Autodesk Inventor part; units mm, degrees
ref_plane "YZ Plane" through (0, 0, 0) normal (1, 0, 0) x (0, 1, 0)
ref_plane "XZ Plane" through (0, 0, 0) normal (0, 1, 0) x (-1, 0, 0)
ref_plane "XY Plane" through (0, 0, 0) normal (0, 0, 1) x (1, 0, 0)
sketch "Sketch1" plane through (0, 0, 0) normal (0, 0, 1) x (1, 0, 0)
  circle A0 centre (0, 0) radius 12.2
  dimension "d0" = 24.4
extrude "Extrusion1" add sketch "Sketch1" along normal blind 34
sketch "Sketch2" plane through (0, 0, 0) normal (0, 0, -1) x (-1, 0, 0)
  circle A0 centre (0, 0) radius 2.5
  dimension "d3" = 5
extrude "Extrusion2" add sketch "Sketch2" along normal blind 8.5
sketch "Sketch3" plane through (0, 0, 0) normal (0, 0, -1) x (-1, 0, 0)
  line L0 (-3.25, -8) -> (3.25, -8) construction
  line L1 (3.25, -8) -> (3.25, -10.5) construction
  line L2 (3.25, -10.5) -> (-3.25, -10.5) construction
  line L3 (-3.25, -10.5) -> (-3.25, -8) construction
  line L4 (0, 0) -> (-3.25, -8) construction
  line L5 (3.25, -8) -> (0, 0) construction
  line L6 (0, 0) -> (0, -8) construction
  line L7 (-7.955, -3.3588) -> (-3.3588, -7.955) construction
  line L8 (-3.3588, -7.955) -> (-5.1265, -9.7227) construction
  line L9 (-5.1265, -9.7227) -> (-9.7227, -5.1265) construction
  line L10 (-9.7227, -5.1265) -> (-7.955, -3.3588) construction
  line L11 (0, 0) -> (-7.955, -3.3588) construction
  line L12 (-3.3588, -7.955) -> (0, 0) construction
  line L13 (0, 0) -> (-5.6569, -5.6569) construction
  circle A0 centre (-2.0637, -9.25) radius 0.5
  circle A1 centre (2.0568, -9.25) radius 0.5
  circle A2 centre (0, -9.25) radius 0.5
  circle A3 centre (-6.5905, -6.5905) radius 0.5
  circle A4 centre (-5.1265, -7.955) radius 0.5
  circle A5 centre (-7.9716, -5.1098) radius 0.5
  dimension "d6" = 2.5
  dimension "d7" = 6.5
  dimension "d8" = 8
  dimension "d9" = 2.5
  dimension "d10" = 6.5
  dimension "d11" = 8
  dimension "d12" = 45
  dimension "d13" = 1
  dimension "d14" = 1
  dimension "d15" = 1
  dimension "d18" = 1
  dimension "d19" = 1
  dimension "d20" = 1
extrude "Extrusion3" add sketch "Sketch3" along normal blind 5 contours A0 | A1 | A2
extrude "Extrusion4" add sketch "Sketch3" along normal blind 5 contours A3 | A4 | A5
properties part number "motor_body"
Geometry check sheet. Reference: the model listing, model coordinates, mm. A direction names the side the tool comes from. Coordinates: 2 decimals unless noted, no trailing zeros. Order: outer loops, then holes, each group sorted by start corner. A loop starts at its lowest first (then second) coordinate and runs counter-clockwise, first axis right, second up. Notation, with made-up numbers: M -28,43.5 L -14,43.5 A18 cw -14,68.5 Z; hole C 18.5,26 d2. An arc over 180 degrees is marked long. One line per question, with ' | ' between items. Start each with the question number.
Item 1: Draft check along Y on faces 4 (the cylindrical face through (-1.95, -8.76, -2.46)), 5 (the cylindrical face through (-12.19, -0.54, 16.76)), 6 (the flat face through (6.6, -6.6, -5)). Enter one of: pulls with the +Y half, pulls with the -Y half, needs draft (parallel to the pull), parting line crosses it, or undercut.
Item 2: Set-up check for faces 1 (the flat face through (5, -8, -5)), 2 (the flat face through (2, -9, -5)), 3 (the cylindrical face through (6.32, -7.01, -2.46)): record each of +Z, -Z, +X, -X, +Y, -Y from which the full face is reachable in a straight line by a thin tool's end or side.
Item 3: Cross-section at B-B on x = 0. Enter the section's corners in (y, z).
Item 4: Cross-section at D-D on z = 21.5. Enter the section's corners in (x, y).
Item 5: Cross-section at C-C on y = -0.5. Enter the section's corners in (x, z), then the cut area to 3 significant figures.
Item 6: Gauge pin test, flat ends, axial feed: pin 1 (6 mm diameter, centred on y = -6, z = 0.5, fed in from -X); pin 2 (5 mm diameter, centred on x = 1, y = 5, fed in from -Z); pin 3 (0.5 mm diameter, centred on x = -2, y = -9.5, fed in from -Z). Record the tip position at first contact, or that the pin passes through.
Item 7: Material ranges on L1, parallel to Z at x = 9.5, y = 2.25; L2, parallel to Y at x = 0.25, z = 1; L3, parallel to Y at x = -1.5, z = 11, recorded low to high. Write a range as [from, to].
Item 8: Cross-section at A-A on z = -4. State how many separate pieces and enclosed holes the cut face has, then the cut area to 3 significant figures.
Findings:
1) face 4: undercut | face 5: parting line crosses it | face 6: needs draft
2) face 1: -Z, +X, -X, +Y, -Y | face 2: -Z, +X, -X, -Y | face 3: -Z
3) outline: M -12.2,0 L -9.75,0 L -9.75,-5 L -8.75,-5 L -8.75,0 L -2.5,0 L -2.5,-8.5 L 2.5,-8.5 L 2.5,0 L 12.2,0 L 12.2,34 L -12.2,34 Z
4) outline: C 0,0 d24.4
5) outline: M -12.19,0 L -2.45,0 L -2.45,-8.5 L 2.45,-8.5 L 2.45,0 L 12.19,0 L 12.19,34 L -12.19,34 Z | area: 871 mm²
6) pin 1: stops at x = -11.83 | pin 2: stops at z = 0 | pin 3: stops at z = -5
7) L1: z = [0, 34] | L2: y = [-12.2, 12.2] | L3: y = [-12.11, 12.11]
8) separate pieces: 7 | enclosed holes: 0 | area: 24.3 mm²
